The model under review builds one solid part; all positions refer to its coordinate system, in mm. A direction names the side the tool comes from. Round coordinates to 2 decimals unless told otherwise and drop trailing zeros. Order: outer loops, then holes, each group sorted by start corner. A loop starts at its lowest first (then second) coordinate and runs counter-clockwise, first axis right, second up. Notation, with made-up numbers: (64.25, -15.75) -> (70.25, -15.75) arc R8 ccw to (70.25, -4.75) -> close; hole circle Ø9 at (-14, 42). An arc over 180 degrees is marked (long way). Return JSON: item names as keys, results as strings. Group by question number.
from build123d import *

# Parameters (mm, degrees)
BASE_FLANGE1_DEPTH = 279.4
SKETCH4_R          = 3.175
TAB1_DEPTH         = 4.7752
SKETCH4_2_R        = 3.175
CUT_EXTRUDE1_DEPTH = 7.62
SKETCH5_R          = 6.35
SKETCH5_R_2        = 2.7813
CUT_EXTRUDE2_DEPTH = 10.16
SKETCH6_R          = 6.35
CUT_EXTRUDE3_DEPTH = 3.429
FILLET1_R          = 12.7
FILLET2_R          = 12.7
SKETCH7_R          = 2.5527
CUT_EXTRUDE4_DEPTH = 7.62


# Sheet-metal steps are written as plain solids
with BuildPart() as part:
    # Sketch1 → Base-Flange1 (new body)
    with BuildSketch(Plane(origin=(0, 0, 0), x_dir=(0, 0, -1), z_dir=(1, 0, 0))):
        with BuildLine():
            Line((0, 0), (0, 63.431940905))
            ThreePointArc((0, 63.431940905), (0.00865484, 63.497680943), (0.034029547, 63.558940905))
            Line((0.034029547, 63.558940905), (229.848055418, 461.608510005))
            ThreePointArc((229.848055418, 461.608510005), (229.869833323, 461.646613437), (229.891277889, 461.684905463))
            Line((229.891277889, 461.684905463), (248.119591573, 494.569653848))
            Line((248.119591573, 494.569653848), (243.943107547, 496.884716746))
            Line((243.943107547, 496.884716746), (225.714793821, 463.999968287))
            ThreePointArc((225.714793821, 463.999968287), (225.713710761, 463.998034347), (225.712610867, 463.996109931))
            Line((225.712610867, 463.996109931), (-4.101414961, 65.946540905))
            ThreePointArc((-4.101414961, 65.946540905), (-4.603834166, 64.733593647), (-4.7752, 63.431940905))
            Line((-4.7752, 63.431940905), (-4.7752, 0))
            Line((-4.7752, 0), (0, 0))
        make_face()
    extrude(amount=-BASE_FLANGE1_DEPTH)

    # Sketch4 → Tab1 (add)
    with BuildSketch(Plane(origin=(0, 11.035159758, 19.907955191), x_dir=(-1, 0, 0), z_dir=(0, -0.48480962024634994, -0.8746197071393886))):
        with Locations((19.05, 534.436130775)):
            Circle(SKETCH4_R)
        with Locations((139.7, 534.436130775)):
            Circle(SKETCH4_R)
        with Locations((260.35, 534.436130775)):
            Circle(SKETCH4_R)
    extrude(amount=-TAB1_DEPTH)

    # Sketch4<2> → Cut-Extrude1 (cut)
    with BuildSketch(Plane(origin=(0, 11.035159758, 19.907955191), x_dir=(-1, 0, 0), z_dir=(0, -0.48480962024634994, -0.8746197071393886))):
        with Locations(Location((19.05, 534.436130775, 0), (0, 0, 90))):
            Circle(SKETCH4_2_R)
        with Locations(Location((139.7, 534.436130775, 0), (0, 0, 90))):
            Circle(SKETCH4_2_R)
        with Locations(Location((260.35, 534.436130775, 0), (0, 0, 90))):
            Circle(SKETCH4_2_R)
    extrude(amount=-CUT_EXTRUDE1_DEPTH, mode=Mode.SUBTRACT)

    # Sketch5 → Cut-Extrude2 (cut)
    with BuildSketch(Plane(origin=(0, 0, 0), x_dir=(-1, 0, 0), z_dir=(0, 0, -1))):
        with Locations((38.1, 34.7472)):
            Circle(SKETCH5_R)
        with Locations((88.9, 34.7472)):
            Circle(SKETCH5_R)
        with Locations((190.5, 34.7472)):
            Circle(SKETCH5_R)
        with Locations((241.3, 34.7472)):
            Circle(SKETCH5_R_2)
    extrude(amount=-CUT_EXTRUDE2_DEPTH, mode=Mode.SUBTRACT)

    # Sketch6 → Cut-Extrude3 (cut)
    with BuildSketch(Plane(origin=(0, 13.350222657, 24.084439216), x_dir=(1, 0, 0), z_dir=(0, 0.48480962024634877, 0.8746197071393893))):
        with Locations(Location((-260.35, 534.436130775, 0), (0, 0, 270))):
            Circle(SKETCH6_R)
        with Locations(Location((-139.7, 534.436130775, 0), (0, 0, 270))):
            Circle(SKETCH6_R)
        with Locations(Location((-19.05, 534.436130775, 0), (0, 0, 270))):
            Circle(SKETCH6_R)
    extrude(amount=-CUT_EXTRUDE3_DEPTH, mode=Mode.SUBTRACT)

    # Fillet1
    fillet1_edges = [part.edges().sort_by_distance(p)[0] for p in [
        (-279.4, 495.727185297, -246.03134956),
    ]]
    fillet(fillet1_edges, radius=FILLET1_R)

    # Fillet2
    fillet2_edges = [part.edges().sort_by_distance(p)[0] for p in [
        (0, 495.727185297, -246.03134956),
    ]]
    fillet(fillet2_edges, radius=FILLET2_R)

    # Sketch7 → Cut-Extrude4 (cut)
    with BuildSketch(Plane(origin=(0, 18.2626, 31.631751078), x_dir=(1, 0, 0), z_dir=(0, 0.5000000000000011, 0.8660254037844382))):
        with Locations(Location((-111.125, 316.624698106, 0), (0, 0, 270))):
            Circle(SKETCH7_R)
        with Locations(Location((-111.125, 253.124698106, 0), (0, 0, 270))):
            Circle(SKETCH7_R)
    extrude(amount=-CUT_EXTRUDE4_DEPTH, mode=Mode.SUBTRACT)


solid = part.part
Item 1: Insertion check: pin 1 Ø4 at (x, z) = (-115, -151.5) entering from -Y; pin 2 Ø5 at (x, y) = (-66, 240) entering from -Z; pin 3 Ø3 at (x, y) = (-56, 210) entering from -Z; pin 4 Ø5 at (x, y) = (-241.3, 34.75) entering from -Z. Each pin has a flat end and moves straight along its axis. Give the tip position at first contact, or say it passes through.
Item 2: Consider section D-D on y = 347. State the section outline as (x, z) points, plus the area to 3 significant figures.
Item 3: For faces 5 (the face through (-138, 31, 0)), 6 (the face through (-21.78, 476.73, -236.69)), 7 (the face through (-3.819, 492.576, -244.246)), list the 3-axis set-ups (+Z, -Z, +X, -X, +Y, -Y) from which the entire face can be reached by the end or side of a thin tool; tool diameter is ignored.
Item 4: Wall thickness on line 1 along Y through (x, z) = (-190.5, 1.95); line 2 along Y through (x, z) = (-88, 1); line 3 along Z through (x, y) = (-115.5, 38): over which ranges is each line inside the solid? List them lowest first.
Item 5: The part is to be moulded in two halves that separate along Y. For faces 1 (the face through (-275.78, 492.4, -244.15)), 2 (the face through (-137.744, 481.551, -240.903)), 3 (the face through (-138, 32, 4.775)), 4 (the face through (-262.78, 474.83, -233.65)), say which applies: +Y half, -Y half, draft (parallel to the pull), parting line (faces both ways), or undercut.
Item 6: Consider section C-C on z = -169.5. State the section outline as (x, y) points, plus the area to 3 significant figures.
Values:
{
 "1": {"pin 1": "y = 322.44", "pin 2": "z = -103.35", "pin 3": "z = -85.45", "pin 4": "through"},
 "2": {"outline": "(-279.4, -163.68) -> (0, -163.68) -> (0, -158.16) -> (-279.4, -158.16) -> close", "area": "1,540 mm^2"},
 "3": {"face 5": "-Z, +X, -X, -Y", "face 6": "none", "face 7": "-Z, +X, +Y"},
 "4": {"line 1": "0 to 28.4, 41.1 to 69.67", "line 2": "0 to 28.46, 41.03 to 71.32", "line 3": "0 to 4.78"},
 "5": {"face 1": "+Y half", "face 2": "-Y half", "face 3": "draft", "face 4": "undercut"},
 "6": {"outline": "(-279.4, 357.08) -> (0, 357.08) -> (0, 366.63) -> (-279.4, 366.63) -> close", "area": "2,670 mm^2"}
}
